```python
from build123d import *

# Parameters (mm, degrees)
SKETCH1_W               = 65
SKETCH1_H               = 94
BOSS_EXTRUDE1_DEPTH     = 2.5
CUT_EXTRUDE1_START      = -1
SKETCH2_R               = 1.5
CUT_EXTRUDE1_DEPTH      = 4.5
LPATTERN1_COUNT         = 3
LPATTERN1_PITCH         = 35
SKETCH3_R               = 1.5
CUT_EXTRUDE2_DEPTH      = 3.5
CUT_EXTRUDE2_DEPTH_BACK = 1


with BuildPart() as part:
    # Sketch1 → Boss-Extrude1 (new body)
    with BuildSketch(Plane.XY):
        Rectangle(SKETCH1_W, SKETCH1_H)
    extrude(amount=BOSS_EXTRUDE1_DEPTH)

    # Sketch2 → Cut-Extrude1 (cut)
    with BuildSketch(Plane.XY.offset(CUT_EXTRUDE1_START)):
        with Locations((-31.25, 37.5)):
            Circle(SKETCH2_R)
        with Locations((31.25, 37.5)):
            Circle(SKETCH2_R)
    cut_extrude1 = extrude(amount=CUT_EXTRUDE1_DEPTH, mode=Mode.SUBTRACT)

    # LPattern1: Cut-Extrude1 ×3
    with Locations(*[(0, -i * LPATTERN1_PITCH, 0) for i in range(1, LPATTERN1_COUNT)]):
        add(cut_extrude1, mode=Mode.SUBTRACT)

    # Sketch3 → Cut-Extrude2 (cut, two sides)
    with BuildSketch(Plane.XY) as cut_extrude2_sk:
        with Locations((0, 45.75)):
            Circle(SKETCH3_R)
    extrude(amount=CUT_EXTRUDE2_DEPTH, mode=Mode.SUBTRACT)
    extrude(cut_extrude2_sk.sketch, amount=-CUT_EXTRUDE2_DEPTH_BACK, mode=Mode.SUBTRACT)


solid = part.part
```
Model file for the job. Use its own axes, mm. Coordinates: 2 decimals unless noted, no trailing zeros. Loops run counter-clockwise (first coordinate to the right, second up) from the corner with the lowest first, then second, coordinate; pieces in that order, holes last. Notation, with made-up numbers: (60.25, 13) - (84.25, 13) arc R27 cw to (84.25, 49) - close; hole circle Ø8 at (-25.75, -36.75). An arc over 180 degrees is marked (long way). Answer as a JSON object with one key per item and string values. Group by question number.
(1) Probe line 1 along Y through (x, z) = (-31.25, 1.8); line 2 along Y through (x, z) = (0, 0.75); line 3 along X through (y, z) = (37.5, 0.9). List the from-to ranges inside material, lowest first.
(2) Flat gauge pin, fed straight in: pin 1 (1.8 mm diameter, centred on x = 31.25, y = 37.5, fed in from +Z). Where does the tip first touch, or does it go through?
(3) Cut at A-A (y = 45.75). Give the cut face in (x, z).
(4) Two-plate mould, pull along X, no slides. Class faces 1 (the face through (0, 1, 2.5)), 2 (the face through (29.75, 37.55, 1.23)), 3 (the face through (-32.5, -15, 1)): released by +X, released by -X, zero draft, split by the parting line, or undercut.
(5) Cut at B-B (x = -31.25). Give the cut face in (y, z), then the cut area to 4 significant figures.
Geometry says:
{
 "1": {"line 1": "y = -47 to -34, -31 to 1, 4 to 36, 39 to 47", "line 2": "y = -47 to 44.25", "line 3": "x = -29.75 to 29.75"},
 "2": {"pin 1": "passes through"},
 "3": {"outline": "(-32.5, 0) - (-1.5, 0) - (-1.5, 2.5) - (-32.5, 2.5) - close; (1.5, 0) - (32.5, 0) - (32.5, 2.5) - (1.5, 2.5) - close"},
 "4": {"face 1": "zero draft", "face 2": "undercut", "face 3": "released by -X"},
 "5": {"outline": "(-47, 0) - (-34, 0) - (-34, 2.5) - (-47, 2.5) - close; (-31, 0) - (1, 0) - (1, 2.5) - (-31, 2.5) - close; (4, 0) - (36, 0) - (36, 2.5) - (4, 2.5) - close; (39, 0) - (47, 0) - (47, 2.5) - (39, 2.5) - close", "area": "212.5 mm^2"}
}
